from build123d import *

# Parameters (mm, degrees)
EXTRUDE_1_DEPTH = 10
SKETCH_2_R      = 17
EXTRUDE_2_DEPTH = 22
MM_1_D          = 7
MM_2_D          = 25


with BuildPart() as part:
    # 草图1 → 凸台-拉伸1 (new body)
    with BuildSketch(Plane(origin=(0, 0, 0), x_dir=(1, 0, 0), z_dir=(0, 1, 0))):
        with BuildLine():
            Line((-12.401209618, 33.9), (-20.986662431, 6.6))
            ThreePointArc((-20.986662431, 6.6), (0, -22), (20.986662431, 6.6))
            Line((20.986662431, 6.6), (12.401209618, 33.9))
            ThreePointArc((12.401209618, 33.9), (0, 43), (-12.401209618, 33.9))
        make_face()
        with BuildLine():
            Line((12.401209618, -33.9), (20.986662431, -6.6))
            ThreePointArc((20.986662431, -6.6), (0, 22), (-20.986662431, -6.6))
            Line((-20.986662431, -6.6), (-12.401209618, -33.9))
            ThreePointArc((-12.401209618, -33.9), (0, -43), (12.401209618, -33.9))
        make_face()
    extrude(amount=EXTRUDE_1_DEPTH)

    # 草图2 → 凸台-拉伸2 (add)
    with BuildSketch(Plane(origin=(0, 10, 0), x_dir=(1, 0, 0), z_dir=(0, 1, 0))):
        with Locations(Location((0, 0, 0), (0, 0, 270))):
            Circle(SKETCH_2_R)
    extrude(amount=EXTRUDE_2_DEPTH)

    # 大小mm 暗销孔1 (through all)
    with Locations(Plane(origin=(0, 10, -30), x_dir=(0, 0, 1), z_dir=(0, 1, 0))):
        with Locations((0, 0), (60, 0)):
            Hole(MM_1_D / 2)

    # 大小mm 暗销孔2 (through all)
    with Locations(Plane.ZX.offset(32)):
        with Locations((0, 0)):
            Hole(MM_2_D / 2)

    # 草图5 → 切除-旋转1 (revolve, cut)
    with BuildSketch(Plane.XY, mode=Mode.PRIVATE) as cut_revolve_1_sk:
        Polygon((0, 22.185045424), (17, 32), (17, 40.592960663), (0, 40.592960663), align=None)
    revolve(cut_revolve_1_sk.sketch.rotate(Axis((0, 32, 0), (0, -1, 0)), 180), axis=Axis((0, 32, 0), (0, -1, 0)), mode=Mode.SUBTRACT)


solid = part.part
Could you check a few things on this model? Use its own coordinates, in mm. A direction names the side the tool comes from. Give positions to 0.01 mm unless a question says otherwise; leave off trailing zeros. Order: outer loops, then holes, each group sorted by start corner. A loop starts at its lowest first (then second) coordinate and runs counter-clockwise, first axis right, second up.
1. Suppose I cut it at D-D (y = 27.5). Write out the boundary of the cut face in (x, z).
Answers below:
outline: circle Ø34 at (0, 0); hole circle Ø25 at (0, 0)
2. Suppose I cut it at A-A (x = 0). Write out the boundary of the cut face in (y, z), plus the area to 3 significant figures.
Answers below:
outline: (0, -43) - (10, -43) - (10, -33.5) - (0, -33.5) - close; (0, -26.5) - (10, -26.5) - (10, -17) - (32, -17) - (29.4, -12.5) - (0, -12.5) - close; (0, 12.5) - (29.4, 12.5) - (32, 17) - (10, 17) - (10, 26.5) - (0, 26.5) - close; (0, 33.5) - (10, 33.5) - (10, 43) - (0, 43) - close
area: 656 mm2
3. Thinking about a two-plate mould opening in Z: for faces 3 (the cylindrical face through (1.05, 4.93, 26.66)), 4 (the flat face through (9, 0, 9)), 5 (the cylindrical face through (0, 5, -43)), 6 (the cylindrical face through (3.755, 14.495, -11.923)), which applies, +Z half, -Z half, draft (parallel to the pull), parting line (faces both ways), or undercut?
Answers below:
face 3: undercut
face 4: draft
face 5: -Z half
face 6: undercut
4. Suppose I cut it at C-C (y = 5). Write out the boundary of the cut face in (x, z), plus the area to 3 significant figures.
Answers below:
outline: (-20.99, -6.6) - (-12.4, -33.9) arc R13 ccw to (12.4, -33.9) - (20.99, -6.6) arc R22 ccw to (20.99, 6.6) - (12.4, 33.9) arc R13 ccw to (-12.4, 33.9) - (-20.99, 6.6) arc R22 ccw to start; hole circle Ø25 at (0, 0); hole circle Ø7 at (0, -30); hole circle Ø7 at (0, 30)
area: 2,160 mm2
5. Suppose I cut it at B-B (z = 0). Write out the boundary of the cut face in (x, y).
Answers below:
outline: (-22, 0) - (-12.5, 0) - (-12.5, 29.4) - (-17, 32) - (-17, 10) - (-22, 10) - close; (12.5, 0) - (22, 0) - (22, 10) - (17, 10) - (17, 32) - (12.5, 29.4) - close
6. For pin 1 (1.5 mm diameter, centred on y = 7.5, z = -33, fed in from +X); pin 2 (12 mm diameter, centred on x = -2, y = 20.5, fed in from +Z); pin 3 (6 mm diameter, centred on x = -14.5, y = 13.5, fed in from +Z), each with a flat end and sliding along its axis, tell me the tip position at first contact or that it passes through.
Answers below:
pin 1: stops at x = 12.92
pin 2: stops at z = 17
pin 3: stops at z = 12.52
7. Which directions (+Z, -Z, +X, -X, +Y, -Y) give clear straight access to the entire face, cutting with the end or side of a thin tool? Please do faces 1 (the flat face through (-16.754, 4.93, 20.059)), 2 (the cylindrical face through (16.855, 20.846, -2.213)).
Answers below:
face 1: +Z, -X, +Y, -Y
face 2: +Y
8. I need wall thicknesses on L1, parallel to X at y = 18, z = 0; L2, parallel to X at y = 6, z = 0; L3, parallel to Z at x = 11.5, y = 27. Which ranges of each line are inside material? Lowest first, please.
Answers below:
L1: x = -17 to -12.5, 12.5 to 17
L2: x = -22 to -12.5, 12.5 to 22
L3: z = -12.52 to -4.9, 4.9 to 12.52
